Could you check a few things on this model? Use its own coordinates, in mm. A direction names the side the tool comes from. Give positions to 0.01 mm unless a question says otherwise; leave off trailing zeros. Loops run counter-clockwise (first coordinate to the right, second up) from the corner with the lowest first, then second, coordinate; pieces in that order, holes last. Notation, with made-up numbers: (84.25, 28) - (121.25, 28) arc R27 cw to (121.25, 46) - close; hole circle Ø10 at (39.25, 61). An arc over 180 degrees is marked (long way). Write each question's results on one line, items separated by ' | '. Start each with the question number.
(1) For pin 1 (3 mm diameter, centred on x = 0, z = 39.5, fed in from -Y); pin 2 (6 mm diameter, centred on y = 2, z = 26, fed in from +X); pin 3 (1.5 mm diameter, centred on y = -8.5, z = 64, fed in from -X), each with a flat end and sliding along its axis, tell me the tip position at first contact or that it passes through.
(2) Suppose I cut it at B-B (z = 72). Please give me the cut outline in (x, y), and give its area (3 significant figures).
(3) Suppose I cut it at C-C (y = 7). Please give me the cut outline in (x, z), and give its area (3 significant figures).
(4) I need wall thicknesses on line 1 (Y direction, x = 16, z = 56); line 2 (Z direction, x = -13, y = 12.5); line 3 (Z direction, x = -10.5, y = 11.5). Which ranges of each line are inside material? Lowest first, please.
(5) On a 3-axis mill with a long thin cutter (end or side, diameter ignored), from which of +Z, -Z, +X, -X, +Y, -Y can I reach the whole of each face in a straight line? I mean faces 4 (the face through (0, 7, 79.5)), 5 (the face through (18.01, 0.07, 56.2)). Say none if no direction works.
(6) If we mould it in two halves opening along X, with no side actions, what happens to faces 1 (the face through (-7.93, -15.762, 56.197)), 2 (the face through (10, -10, 58)), 3 (the face through (-3.47, -15.62, 14.79))? For each: released by +X, released by -X, zero draft, split by the parting line, or undercut.
(7) Suppose I cut it at A-A (x = 0). Please give me the cut outline in (y, z).
(8) Suppose I cut it at D-D (x = -4.5). Please give me the cut outline in (y, z), and give its area (3 significant figures).
from build123d import *

# Parameters (mm, degrees)
SKETCH1_R                    = 16
BOSS_EXTRUDE1_DEPTH          = 30
SKETCH2_R                    = 18.5
BOSS_EXTRUDE2_DEPTH          = 28
SKETCH3_R                    = 13.255383993
BOSS_EXTRUDE3_DEPTH          = 6
SKETCH4_R                    = 3
BOSS_EXTRUDE4_DEPTH          = 15.5
F_3_0_3_DIAMETER_HOLE2_D     = 3
F_3_0_3_DIAMETER_HOLE2_DEPTH = 3.556
F_3_0_3_DIAMETER_HOLE2_TIP   = 0.901290929
F_3_0_3_DIAMETER_HOLE1_D     = 3
F_3_0_3_DIAMETER_HOLE1_DEPTH = 3.499993
F_3_0_3_DIAMETER_HOLE1_TIP   = 0.901290929


with BuildPart() as part:
    # Sketch1 → Boss-Extrude1 (new body)
    with BuildSketch(Plane.XY):
        Circle(SKETCH1_R)
    extrude(amount=BOSS_EXTRUDE1_DEPTH)

    # Sketch2 → Boss-Extrude2 (add)
    with BuildSketch(Plane.XY.offset(30)):
        Circle(SKETCH2_R)
    extrude(amount=BOSS_EXTRUDE2_DEPTH)

    # Sketch3 → Boss-Extrude3 (add)
    with BuildSketch(Plane.XY.offset(58)):
        Circle(SKETCH3_R)
    extrude(amount=BOSS_EXTRUDE3_DEPTH)

    # Sketch4 → Boss-Extrude4 (add)
    with BuildSketch(Plane.XY.offset(64)):
        with Locations((0, 7)):
            Circle(SKETCH4_R)
    extrude(amount=BOSS_EXTRUDE4_DEPTH)

    # Ø3.0 (3) Diameter Hole2
    with Locations(Plane.XY.offset(58)):
        with Locations((-8.079199421, 13.993583881), (-16.51, 0), (8.255, -14.298079416), (-8.255, -14.298079416), (8.255, 14.298079416), (16.51, 0)):
            Hole(F_3_0_3_DIAMETER_HOLE2_D / 2, depth=F_3_0_3_DIAMETER_HOLE2_DEPTH)
            with Locations((0, 0, -(F_3_0_3_DIAMETER_HOLE2_DEPTH + F_3_0_3_DIAMETER_HOLE2_TIP / 2))):  # 118° drill point
                Cone(0, F_3_0_3_DIAMETER_HOLE2_D / 2, F_3_0_3_DIAMETER_HOLE2_TIP, mode=Mode.SUBTRACT)

    # Ø3.0 (3) Diameter Hole1
    with Locations(Plane.XY.offset(58)):
        with Locations((-16.51, 0), (8.255, -14.298079416), (16.51, 0), (8.255, 14.298079416)):
            Hole(F_3_0_3_DIAMETER_HOLE1_D / 2, depth=F_3_0_3_DIAMETER_HOLE1_DEPTH)
            with Locations((0, 0, -(F_3_0_3_DIAMETER_HOLE1_DEPTH + F_3_0_3_DIAMETER_HOLE1_TIP / 2))):  # 118° drill point
                Cone(0, F_3_0_3_DIAMETER_HOLE1_D / 2, F_3_0_3_DIAMETER_HOLE1_TIP, mode=Mode.SUBTRACT)


solid = part.part
Output values:
1) pin 1: y = -18.5 | pin 2: x = 16 | pin 3: x = -10.75
2) outline: circle Ø6 at (0, 7) | area: 28.3 mm2
3) outline: (-17.12, 30) - (-14.39, 30) - (-14.39, 0) - (14.39, 0) - (14.39, 30) - (17.12, 30) - (17.12, 58) - (11.26, 58) - (11.26, 64) - (3, 64) - (3, 79.5) - (-3, 79.5) - (-3, 64) - (-11.26, 64) - (-11.26, 58) - (-17.12, 58) - close | area: 2,050 mm2
4) line 1: -9.29 to -1.41, 1.41 to 9.29 | line 2: 30 to 58 | line 3: 0 to 58
5) face 4: +Z, +X, -X, +Y, -Y | face 5: +Z
6) face 1: undercut | face 2: zero draft | face 3: split by the parting line
7) outline: (-18.5, 30) - (-16, 30) - (-16, 0) - (16, 0) - (16, 30) - (18.5, 30) - (18.5, 58) - (13.26, 58) - (13.26, 64) - (10, 64) - (10, 79.5) - (4, 79.5) - (4, 64) - (-13.26, 64) - (-13.26, 58) - (-18.5, 58) - close
8) outline: (-17.94, 30) - (-15.35, 30) - (-15.35, 0) - (15.35, 0) - (15.35, 30) - (17.94, 30) - (17.94, 58) - (12.47, 58) - (12.47, 64) - (-12.47, 64) - (-12.47, 58) - (-17.94, 58) - close | area: 2,080 mm2
